Read the model definition and answer for the solid it produces. Units are mm, in the model's axes. Face numbers are marked on the shaded views. Give positions to 0.01 mm unless a question says otherwise; leave off trailing zeros. Order: outer loops, then holes, each group sorted by start corner. A loop starts at its lowest first (then second) coordinate and runs counter-clockwise, first axis right, second up.
Item 1: A cutting plane is placed at A-A (z = 3). Write down the section's boundary in (x, y).
Item 2: Given pin 1 Ø1.6 at (x, y) = (-5, -7) entering from -Z; pin 2 Ø2 at (x, y) = (2, -17.5) entering from -Z, each flat-ended and moving along its own axis, determine where each tip first touches the part or whether it passes through.
Item 3: A cutting plane is placed at C-C (y = -27). Write down the section's boundary in (x, z).
Item 4: A cutting plane is placed at B-B (x = -1.25). Write down the section's boundary in (y, z), plus the area to 3 significant figures.
Item 5: A cutting plane is placed at D-D (x = -5). Write down the section's boundary in (y, z), plus the area to 3 significant figures.
Item 6: Find the intervals of material crossed by line 1 along Y through (x, z) = (-2, 2.75); line 2 along Z through (x, y) = (0.25, -12), in increasing order.
Item 7: The mould has two halves that part along Y. Classify the marked faces 1, 2 and 3: +Y half, -Y half, draft (parallel to the pull), parting line (faces both ways), or undercut.
from build123d import *

# Parameters (mm, degrees)
ESQUISSE1_W             = 20
ESQUISSE1_H             = 51
EXTRUSION1_DEPTH        = 9
ESQUISSE3_W             = 7
ESQUISSE3_H             = 20
ENL_V_MAT_EXTRU_1_DEPTH = 2
ENL_V_MAT_EXTRU_2_REACH = 52.881
ESQUISSE4_W             = 5
ESQUISSE4_H             = 2


with BuildPart() as part:
    # Esquisse1 → Extrusion1 (new body)
    with BuildSketch(Plane.XY):
        with Locations((-5.903123543, -20.411538462)):
            Rectangle(ESQUISSE1_W, ESQUISSE1_H)
    extrude(amount=EXTRUSION1_DEPTH)

    # Esquisse3 → Enlèv. mat.-Extru.1 (cut)
    with BuildSketch(Plane(origin=(0, 0, 0), x_dir=(-1, 0, 0), z_dir=(0, 0, -1))):
        with Locations((-0.596876457, -17.911538462)):
            Rectangle(ESQUISSE3_W, ESQUISSE3_H)
    extrude(amount=-ENL_V_MAT_EXTRU_1_DEPTH, mode=Mode.SUBTRACT)

    # Esquisse4 → Enlèv. mat.-Extru.2 (cut, up to next)
    with BuildSketch(Plane(origin=(4.096876457, 0, 0), x_dir=(0, 0, -1), z_dir=(1, 0, 0)), mode=Mode.PRIVATE) as enl_v_mat_extru_2_sk1:
        with Locations((-2.5, -6.911538462)):
            Rectangle(ESQUISSE4_W, ESQUISSE4_H)
    enl_v_mat_extru_2_tool1 = extrude(enl_v_mat_extru_2_sk1.sketch, amount=-ENL_V_MAT_EXTRU_2_REACH, mode=Mode.PRIVATE) & part.part
    add(enl_v_mat_extru_2_tool1.solids().sort_by_distance((4.096876, -6.911538, 2.5))[0], mode=Mode.SUBTRACT)


solid = part.part
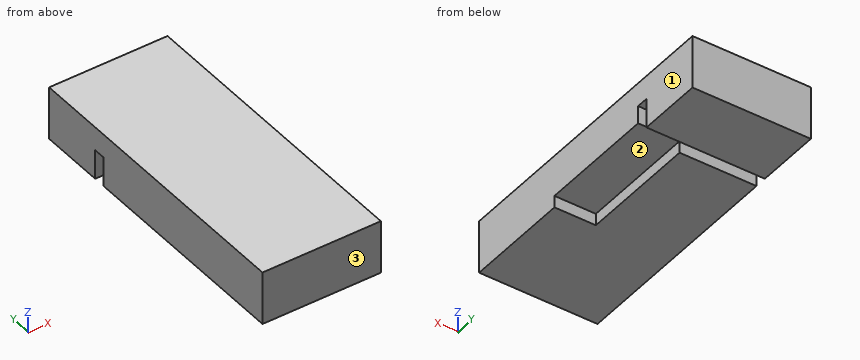
Response values:
1. outline: (-15.9, -45.91) - (4.1, -45.91) - (4.1, -7.91) - (-15.9, -7.91) - close; (-15.9, -5.91) - (4.1, -5.91) - (4.1, 5.09) - (-15.9, 5.09) - close
2. pin 1: stops at z = 5
2. pin 2: stops at z = 2
3. outline: (-15.9, 0) - (-2.9, 0) - (-2.9, 2) - (4.1, 2) - (4.1, 9) - (-15.9, 9) - close
4. outline: (-45.91, 0) - (-27.91, 0) - (-27.91, 2) - (-7.91, 2) - (-7.91, 5) - (-5.91, 5) - (-5.91, 0) - (5.09, 0) - (5.09, 9) - (-45.91, 9) - close
4. area: 409 mm2
5. outline: (-45.91, 0) - (-7.91, 0) - (-7.91, 5) - (-5.91, 5) - (-5.91, 0) - (5.09, 0) - (5.09, 9) - (-45.91, 9) - close
5. area: 449 mm2
6. line 1: y = -45.91 to -7.91, -5.91 to 5.09
6. line 2: z = 2 to 9
7. face 1: draft
7. face 2: undercut
7. face 3: -Y half
